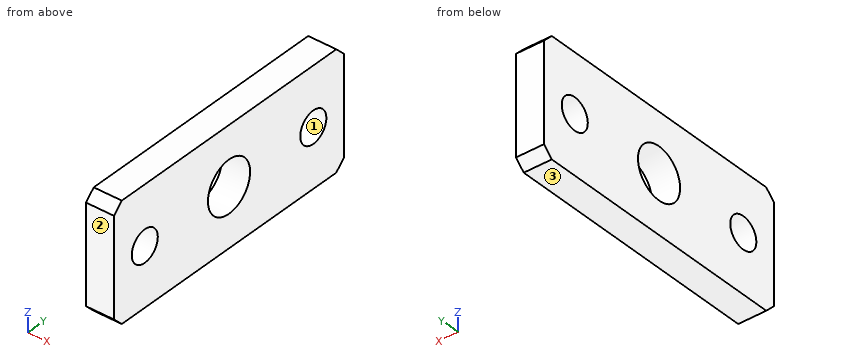
from build123d import *

# Parameters (mm, degrees)
SKETCH1_W                  = 25
SKETCH1_H                  = 60
BOSS_EXTRUDE1_DEPTH        = 6
F_11_0_11_DIAMETER_HOLE1_D = 11
M8X1_25_TAPPED_HOLE1_D     = 6.8
CHAMFER1_SIZE              = 2


with BuildPart() as part:
    # Sketch1 → Boss-Extrude1 (new body)
    with BuildSketch(Plane(origin=(0, 0, 0), x_dir=(0, 0, -1), z_dir=(1, 0, 0))):
        with Locations((12.5, 0)):
            Rectangle(SKETCH1_W, SKETCH1_H)
    extrude(amount=-BOSS_EXTRUDE1_DEPTH)

    # Ø11.0 (11) Diameter Hole1 (through all)
    with Locations(Plane(origin=(0, 0, 0), x_dir=(0, 0, -1), z_dir=(1, 0, 0))):
        with Locations((12.5, 0)):
            Hole(F_11_0_11_DIAMETER_HOLE1_D / 2)

    # M8x1.25 Tapped Hole1 (through all)
    with Locations(Plane(origin=(0, 0, 0), x_dir=(0, 0, -1), z_dir=(1, 0, 0))):
        with Locations((12.5, 22), (12.5, -22)):
            Hole(M8X1_25_TAPPED_HOLE1_D / 2)

    # Chamfer1
    chamfer1_edges = [part.edges().sort_by_distance(p)[0] for p in [
        (-3, 30, 0),
        (-3, 30, -25),
        (-3, -30, -25),
        (-3, -30, 0),
    ]]
    chamfer(chamfer1_edges, length=CHAMFER1_SIZE)


solid = part.part
Check sheet for the modelled part. Datum: model origin and axes. Units: mm. Face numbers are marked on the shaded views. Round coordinates to 2 decimals unless told otherwise and drop trailing zeros. Loops run counter-clockwise (first coordinate to the right, second up) from the corner with the lowest first, then second, coordinate; pieces in that order, holes last.
1. Sectioned sample at C-C on x = -2.75. Record the boundary of the cut face in (y, z).
2. Mould release check, pull along Y, two halves, no side actions. Record for the marked faces 1, 2 and 3: released by +Y, released by -Y, zero draft, split by the parting line, or undercut.
3. Sectioned sample at A-A on z = -12.5. Record the boundary of the cut face in (x, y), and give its area (3 significant figures).
4. Sectioned sample at B-B on y = 0. Record the boundary of the cut face in (x, z).
5. Scan lines: probe 1 along Y at (x, z) = (-2.55, -12.5); probe 2 along Y at (x, z) = (-1.2, -15); probe 3 along Z at (x, y) = (-1.25, -25). Record each from-to range of solid material in increasing order.
6. Sectioned sample at D-D on z = -8.25. Record the boundary of the cut face in (x, y).
Recorded:
1. outline: (-30, -23) - (-28, -25) - (28, -25) - (30, -23) - (30, -2) - (28, 0) - (-28, 0) - (-30, -2) - close; hole circle Ø6.8 at (-22, -12.5); hole circle Ø11 at (0, -12.5); hole circle Ø6.8 at (22, -12.5)
2. face 1: undercut
2. face 2: released by -Y
2. face 3: zero draft
3. outline: (-6, -30) - (0, -30) - (0, -25.4) - (-6, -25.4) - close; (-6, -18.6) - (0, -18.6) - (0, -5.5) - (-6, -5.5) - close; (-6, 5.5) - (0, 5.5) - (0, 18.6) - (-6, 18.6) - close; (-6, 25.4) - (0, 25.4) - (0, 30) - (-6, 30) - close
3. area: 212 mm2
4. outline: (-6, -25) - (0, -25) - (0, -18) - (-6, -18) - close; (-6, -7) - (0, -7) - (0, 0) - (-6, 0) - close
5. probe 1: y = -30 to -25.4, -18.6 to -5.5, 5.5 to 18.6, 25.4 to 30
5. probe 2: y = -30 to -24.3, -19.7 to -4.9, 4.9 to 19.7, 24.3 to 30
5. probe 3: z = -25 to -14.1, -10.9 to 0
6. outline: (-6, -30) - (0, -30) - (0, -3.49) - (-6, -3.49) - close; (-6, 3.49) - (0, 3.49) - (0, 30) - (-6, 30) - close
